Build history of the part. All positions in model axes, mm. Face numbers are marked on the shaded views. A direction names the side the tool comes from. Give positions to 0.01 mm unless a question says otherwise; leave off trailing zeros. Order: outer loops, then holes, each group sorted by start corner. A loop starts at its lowest first (then second) coordinate and runs counter-clockwise, first axis right, second up. Notation, with made-up numbers: (50, -22) - (105, -22) arc R25 cw to (105, -10) - close; hole circle Ø2 at (14, 46). An arc over 180 degrees is marked (long way). Answer in a Markdown table with one row per item.
```python
from build123d import *

# Parameters (mm, degrees)
SKETCH_2_W          = 100
SKETCH_2_H          = 100
EXTRUDE_1_DEPTH     = 4
EXTRUDE_1_2_DEPTH   = 76
EXTRUDE_2_DEPTH     = 2
CUT_EXTRUDE_1_DEPTH = 70.5
SKETCH_6_R          = 5.5
CUT_EXTRUDE_2_DEPTH = 5
FILLET_1_R          = 10


with BuildPart() as part:
    # Эскиз2 → Extrude 1 (new body)
    with BuildSketch(Plane(origin=(0, 0, 0), x_dir=(1, 0, 0), z_dir=(0, 1, 0))):
        Rectangle(SKETCH_2_W, SKETCH_2_H)
    extrude(amount=EXTRUDE_1_DEPTH)

    # Эскиз3 → Extrude 1 2 (add)
    with BuildSketch(Plane(origin=(0, 4, 0), x_dir=(1, 0, 0), z_dir=(0, 1, 0))):
        with BuildLine():
            Line((-15.5, -15), (-15.5, 14))
            ThreePointArc((-15.5, 14), (-15.207106781, 14.707106781), (-14.5, 15))
            Line((-14.5, 15), (14.5, 15))
            ThreePointArc((14.5, 15), (15.207106781, 14.707106781), (15.5, 14))
            Line((15.5, 14), (15.5, -15))
            Line((15.5, -15), (19.5, -15))
            Line((19.5, -15), (19.5, 14))
            ThreePointArc((19.5, 14), (18.035533906, 17.535533906), (14.5, 19))
            Line((14.5, 19), (-14.5, 19))
            ThreePointArc((-14.5, 19), (-18.035533906, 17.535533906), (-19.5, 14))
            Line((-19.5, 14), (-19.5, -15))
            Line((-19.5, -15), (-15.5, -15))
        make_face()
    extrude(amount=EXTRUDE_1_2_DEPTH)

    # Эскиз4 → Бобышка-Вытянуть2 (add, symmetric)
    with BuildSketch(Plane(origin=(0, 0, 0), x_dir=(0, 0, -1), z_dir=(1, 0, 0))):
        Polygon((19, 49.033320997), (45, 4), (19, 4), align=None)
    extrude(amount=EXTRUDE_2_DEPTH, both=True)

    # Эскиз5 → Вырез-Вытянуть1 (cut, through all)
    with BuildSketch(Plane(origin=(19.5, 0, 0), x_dir=(0, 0, -1), z_dir=(1, 0, 0))):
        with BuildLine():
            Line((5, 68), (5, 56))
            ThreePointArc((5, 56), (0, 51), (-5, 56))
            Line((-5, 56), (-5, 68))
            ThreePointArc((-5, 68), (0, 73), (5, 68))
        make_face()
        with BuildLine():
            Line((5, 28), (5, 16))
            ThreePointArc((5, 16), (0, 11), (-5, 16))
            Line((-5, 16), (-5, 28))
            ThreePointArc((-5, 28), (0, 33), (5, 28))
        make_face()
    extrude(amount=-CUT_EXTRUDE_1_DEPTH, mode=Mode.SUBTRACT)

    # Эскиз6 → Вырез-Вытянуть2 (cut, through all)
    with BuildSketch(Plane(origin=(0, 4, 0), x_dir=(1, 0, 0), z_dir=(0, 1, 0))):
        with Locations(Location((-35, 35, 0), (0, 0, 270))):  # turned: the seam where the file's is
            Circle(SKETCH_6_R)
        with Locations(Location((-35, -35, 0), (0, 0, 270))):  # turned: the seam where the file's is
            Circle(SKETCH_6_R)
        with Locations(Location((35, 35, 0), (0, 0, 270))):  # turned: the seam where the file's is
            Circle(SKETCH_6_R)
        with Locations(Location((35, -35, 0), (0, 0, 270))):  # turned: the seam where the file's is
            Circle(SKETCH_6_R)
    extrude(amount=-CUT_EXTRUDE_2_DEPTH, mode=Mode.SUBTRACT)

    # Скругление1
    fillet_1_edges = [part.edges().sort_by_distance(p)[0] for p in [
        (50, 2, 50),
        (-50, 2, 50),
        (-50, 2, -50),
        (50, 2, -50),
    ]]
    fillet(fillet_1_edges, radius=FILLET_1_R)


solid = part.part
```
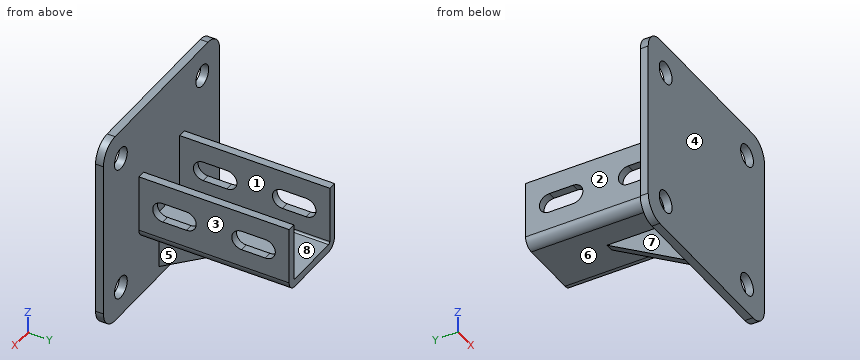
1. Cut at B-B on y = 59. Write the cut outline in (x, z).
Check result:
| item | result |
|---|---|
| outline | (-19.5, -14) arc R5 ccw to (-14.5, -19) - (14.5, -19) arc R5 ccw to (19.5, -14) - (19.5, -5) - (15.5, -5) - (15.5, -14) arc R1 cw to (14.5, -15) - (-14.5, -15) arc R1 cw to (-15.5, -14) - (-15.5, -5) - (-19.5, -5) - close; (-19.5, 5) - (-15.5, 5) - (-15.5, 15) - (-19.5, 15) - close; (15.5, 5) - (19.5, 5) - (19.5, 15) - (15.5, 15) - close |
2. Which spindle directions (+Z, -Z, +X, -X, +Y, -Y) get a long thin tool onto all of the face, cutting with end or side? Do the marked faces 1, 2, 3 and 4. Say none if no direction does.
Check result:
| item | result |
|---|---|
| face 1 | +Z, +Y |
| face 2 | +Z, -Z, -X, +Y |
| face 3 | +Z, -Z, +X, +Y |
| face 4 | +Z, -Z, +X, -X, -Y |
3. Two-plate mould, pull along X, no slides. Class the marked faces 5, 6, 7 and 8: +X half, -X half, draft (parallel to the pull), parting line (faces both ways), or undercut.
Check result:
| item | result |
|---|---|
| face 5 | +X half |
| face 6 | draft |
| face 7 | -X half |
| face 8 | undercut |
4. Drop flat-ended pins along their axis: P1, Ø1.2, axis at x = 18, y = 61, coming from the +Z side; P2, Ø6, axis at x = 19, y = 62, coming from the -Z side; P3, Ø8.5, axis at y = 56, z = -5.5, coming from the +X side; P4, Ø9, axis at x = 35, z = -35, coming from the +Y side. Give the stop position or say it passes through.
Check result:
| item | result |
|---|---|
| P1 | stops at z = 15 |
| P2 | stops at z = -18.77 |
| P3 | stops at x = 19.5 |
| P4 | passes through |
5. Cut at A-A on z = 35. Write the cut outline in (x, y), and give its area (3 significant figures).
Check result:
| item | result |
|---|---|
| outline | (-50, 0) - (-40.5, 0) - (-40.5, 4) - (-50, 4) - close; (-29.5, 0) - (29.5, 0) - (29.5, 4) - (-29.5, 4) - close; (40.5, 0) - (50, 0) - (50, 4) - (40.5, 4) - close |
| area | 312 mm² |
6. Probe line 1 (X direction, y = 1.4, z = 35); line 2 (X direction, y = 36, z = 13.5); line 3 (Y direction, x = 42, z = -15). List the from-to ranges inside material, lowest first.
Check result:
| item | result |
|---|---|
| line 1 | x = -50 to -40.5, -29.5 to 29.5, 40.5 to 50 |
| line 2 | x = -19.5 to -15.5, 15.5 to 19.5 |
| line 3 | y = 0 to 4 |
7. Cut at D-D on x = -11.5. Write the cut outline in (y, z), and give its area (3 significant figures).
Check result:
| item | result |
|---|---|
| outline | (0, -50) - (4, -50) - (4, -19) - (80, -19) - (80, -15) - (4, -15) - (4, 50) - (0, 50) - close |
| area | 704 mm² |
8. Cut at C-C on x = -35. Write the cut outline in (y, z), and give its area (3 significant figures).
Check result:
| item | result |
|---|---|
| outline | (0, -50) - (4, -50) - (4, -40.5) - (0, -40.5) - close; (0, -29.5) - (4, -29.5) - (4, 29.5) - (0, 29.5) - close; (0, 40.5) - (4, 40.5) - (4, 50) - (0, 50) - close |
| area | 312 mm² |
